Design review of the part built by this model. Coordinates are the model's own, in mm. A direction names the side the tool comes from. Give positions to 0.01 mm unless a question says otherwise; leave off trailing zeros. Loops run counter-clockwise (first coordinate to the right, second up) from the corner with the lowest first, then second, coordinate; pieces in that order, holes last.
from build123d import *

# Parameters (mm, degrees)
BOSS_EXTRUDE1_DEPTH     = 39
CUT_EXTRUDE1_DEPTH      = 53.796769788
CUT_EXTRUDE2_DEPTH      = 58.361049502
CUT_EXTRUDE2_DEPTH_BACK = 10
SKETCH3_R               = 4
CHAMFER1_SIZE           = 1.5


with BuildPart() as part:
    # Sketch1 → Boss-Extrude1 (new, symmetric)
    with BuildSketch(Plane(origin=(0, 0, 0), x_dir=(0, 0, -1), z_dir=(1, 0, 0))):
        with BuildLine():
            Line((-1.5, 0), (-1.5, -7.67))
            ThreePointArc((-1.5, -7.67), (-1.939339828, -8.730660172), (-3, -9.17))
            Line((-3, -9.17), (-19.2, -9.17))
            ThreePointArc((-19.2, -9.17), (-20.260660172, -8.730660172), (-20.7, -7.67))
            Line((-20.7, -7.67), (-20.7, -1.17))
            Line((-20.7, -1.17), (-16.95, -3.335063509))
            ThreePointArc((-16.95, -3.335063509), (-15.45, -3.335063509), (-14.7, -2.036025404))
            Line((-14.7, -2.036025404), (-14.7, 22.83))
            Line((-14.7, 22.83), (3.3, 22.83))
            Line((3.3, 22.83), (3.3, 15.83))
            Line((3.3, 15.83), (5.087630389, 17.33))
            Line((5.087630389, 17.33), (7.087630389, 17.33))
            Line((7.087630389, 17.33), (8.875260778, 15.83))
            Line((8.875260778, 15.83), (25.8, 15.83))
            Line((25.8, 15.83), (27.3, 14.33))
            Line((27.3, 14.33), (27.3, 3))
            ThreePointArc((27.3, 3), (26.860660172, 1.939339828), (25.8, 1.5))
            Line((25.8, 1.5), (0, 1.5))
            ThreePointArc((0, 1.5), (-1.060660172, 1.060660172), (-1.5, 0))
        make_face()
    extrude(amount=BOSS_EXTRUDE1_DEPTH, both=True)

    # Sketch2 → Cut-Extrude1 (cut, symmetric)
    with BuildSketch(Plane.XY):
        Polygon((-39, 22.83), (-35.438170518, 22.83), (-35.438170518, 12.163333333), (-39, 4.163333333), align=None)
    cut_extrude1 = extrude(amount=CUT_EXTRUDE1_DEPTH, both=True, mode=Mode.SUBTRACT)

    # Mirror2: Cut-Extrude1 across plane
    add(cut_extrude1.mirror(Plane(origin=(0, 0, 0), x_dir=(0, 0, 1), z_dir=(1, 0, 0))), mode=Mode.SUBTRACT)

    # Sketch3 → Cut-Extrude2 (cut, two sides: drawn at the far end of the back side and taken through both)
    with BuildSketch(Plane(origin=(0, 22.83, 0), x_dir=(1, 0, 0), z_dir=(0, 1, 0)).offset(-CUT_EXTRUDE2_DEPTH_BACK)):
        with Locations(Location((23.438170518, -5.7, 0), (0, 0, 90))):
            Circle(SKETCH3_R)
        with Locations(Location((0, -5.7, 0), (0, 0, 90))):
            Circle(SKETCH3_R)
        with Locations(Location((-23.438170518, -5.7, 0), (0, 0, 90))):
            Circle(SKETCH3_R)
    extrude(amount=CUT_EXTRUDE2_DEPTH + CUT_EXTRUDE2_DEPTH_BACK, mode=Mode.SUBTRACT)

    # Chamfer1
    chamfer1_edges = [part.edges().sort_by_distance(p)[0] for p in [
        (23.438170518, 22.83, 9.7),
        (0, 22.83, 9.7),
        (-23.438170518, 22.83, 9.7),
    ]]
    chamfer(chamfer1_edges, length=CHAMFER1_SIZE)


solid = part.part
Q1. Tool access review of faces 1 (the face through (24.97, 17.02, 2.005)), 2 (the face through (0.55, -8.74, 20.25)), 3 (the face through (0, 19, -3.3)), 4 (the face through (0, 17.33, -6)): name each direction out of +Z, -Z, +X, -X, +Y, -Y from which nothing blocks a thin tool from reaching the whole face with its end or side.
Results:
face 1: +Y
face 2: +Z, +X, -X, -Y
face 3: +X, -X, +Y
face 4: -Z, +X, -X, +Y
Q2. Take a section at B-B (x = -16.5). Give the boundary of the cut face in (y, z), plus the area to 3 significant figures.
Results:
outline: (-9.17, 3) arc R1.5 ccw to (-7.67, 1.5) - (0, 1.5) arc R1.5 cw to (1.5, 0) - (1.5, -25.8) arc R1.5 ccw to (3, -27.3) - (14.33, -27.3) - (15.83, -25.8) - (15.83, -8.88) - (17.33, -7.09) - (17.33, -5.09) - (15.83, -3.3) - (22.83, -3.3) - (22.83, 14.7) - (-2.04, 14.7) arc R1.5 cw to (-3.34, 16.95) - (-1.17, 20.7) - (-7.67, 20.7) arc R1.5 ccw to (-9.17, 19.2) - close
area: 911 mm2
Q3. Take a section at C-C (z = 5.7). Give the boundary of the cut face in (x, y), plus the area to 3 significant figures.
Results:
outline: (-39, -9.17) - (39, -9.17) - (39, 4.16) - (35.44, 12.16) - (35.44, 22.83) - (28.94, 22.83) - (27.44, 21.33) - (27.44, 12.83) - (19.44, 12.83) - (19.44, 21.33) - (17.94, 22.83) - (5.5, 22.83) - (4, 21.33) - (4, 12.83) - (-4, 12.83) - (-4, 21.33) - (-5.5, 22.83) - (-17.94, 22.83) - (-19.44, 21.33) - (-19.44, 12.83) - (-27.44, 12.83) - (-27.44, 21.33) - (-28.94, 22.83) - (-35.44, 22.83) - (-35.44, 12.16) - (-39, 4.16) - close
area: 2,140 mm2
Q4. Take a section at D-D (x = 0). Give the boundary of the cut face in (y, z).
Results:
outline: (-9.17, 3) arc R1.5 ccw to (-7.67, 1.5) - (0, 1.5) arc R1.5 cw to (1.5, 0) - (1.5, -25.8) arc R1.5 ccw to (3, -27.3) - (14.33, -27.3) - (15.83, -25.8) - (15.83, -8.88) - (17.33, -7.09) - (17.33, -5.09) - (15.83, -3.3) - (22.83, -3.3) - (22.83, 0.2) - (21.33, 1.7) - (12.83, 1.7) - (12.83, 9.7) - (21.33, 9.7) - (22.83, 11.2) - (22.83, 14.7) - (-2.04, 14.7) arc R1.5 cw to (-3.34, 16.95) - (-1.17, 20.7) - (-7.67, 20.7) arc R1.5 ccw to (-9.17, 19.2) - close
Q5. Take a section at A-A (z = -21.5). Give the boundary of the cut face in (x, y).
Results:
outline: (-39, 1.5) - (39, 1.5) - (39, 4.16) - (35.44, 12.16) - (35.44, 15.83) - (-35.44, 15.83) - (-35.44, 12.16) - (-39, 4.16) - close
Q6. Draft analysis for pull direction X (two halves, no side actions). For faces 5 (the face through (0.55, 1.07, 1.05)), 6 (the face through (-35.438, 16, -1)), 7 (the face through (-23, 12.83, 6)), 8 (the face through (23, 12.83, 6)), state which applies: pulls with the +X half, pulls with the -X half, needs draft (parallel to the pull), parting line crosses it, or undercut.
Results:
face 5: needs draft
face 6: pulls with the -X half
face 7: undercut
face 8: undercut
Q7. Insertion check: pin 1 (1 mm diameter, centred on x = 13, z = -5.5, fed in from -Y); pin 2 (11.5 mm diameter, centred on y = 17, z = 1, fed in from -X); pin 3 (4 mm diameter, centred on y = 12, z = 13.5, fed in from -X). Each pin has a flat end and moves straight along its axis. Give the tip position at first contact, or say it passes through.
Results:
pin 1: stops at y = 1.5
pin 2: stops at x = -35.84
pin 3: stops at x = -36.4
Q8. Wall thickness on line 1 (X direction, y = 17.5, z = 5.7); line 2 (X direction, y = 18, z = 3); line 3 (Z direction, x = 6, y = 14): over which ranges is each line inside the solid? List them lowest first.
Results:
line 1: x = -35.44 to -27.44, -19.44 to -4, 4 to 19.44, 27.44 to 35.44
line 2: x = -35.44 to -26.39, -20.49 to -2.95, 2.95 to 20.49, 26.39 to 35.44
line 3: z = -27.3 to 14.7
